```python
from build123d import *

# Parameters (mm, degrees)
SKICA1_W                                  = 49.2698
SKICA1_H                                  = 40
P_IDAT_VYSUNUT_M1_DEPTH                   = 2
ZKOSEN_1_SIZE                             = 0.5
SKICA4_W                                  = 63.2698
SKICA4_H                                  = 46
P_IDAT_VYSUNUT_M2_DEPTH                   = 2
KU_ELOV_ZAHLOUBEN_PRO_M3_ROUBU_SE_2_COUNT = 2
KU_ELOV_ZAHLOUBEN_PRO_M3_ROUBU_SE_2_PITCH = 66.661315559
F_3_4_3_4_PR_M_R_D_RY1_D                  = 3.4
F_3_4_3_4_PR_M_R_D_RY1_DEPTH              = 2
ODEBRAT_VYSUNUT_M1_DEPTH                  = 2
F_3_5_3_5_PR_M_R_D_RY1_D                  = 3.5
F_3_5_3_5_PR_M_R_D_RY1_DEPTH              = 4
F_4_5_4_5_PR_M_R_D_RY1_D                  = 4.5
F_4_5_4_5_PR_M_R_D_RY1_DEPTH              = 4
ZKOSEN_2_SIZE                             = 0.5


with BuildPart() as part:
    # Skica1 → Přidat vysunutím1 (new body)
    with BuildSketch(Plane.XY):
        with Locations((-294.244757855, 0)):
            Rectangle(SKICA1_W, SKICA1_H)
    extrude(amount=-P_IDAT_VYSUNUT_M1_DEPTH)

    # Zkosení1
    zkosen_1_edges = [part.edges().sort_by_distance(p)[0] for p in [
        (-269.609857855, 0, -2),
        (-294.244757855, 20, -2),
        (-318.879657855, 0, -2),
        (-294.244757855, -20, -2),
    ]]
    chamfer(zkosen_1_edges, length=ZKOSEN_1_SIZE)

    # Skica3 → Odebrat rotací2 (revolve, cut)
    with BuildSketch(Plane(origin=(0, -13.1125, 0), x_dir=(-1, 0, 0), z_dir=(0, -1, 0))):
        Polygon((273.341908662, 2), (276.609857855, 0.113248654), (276.609857855, 2), align=None)
    revolve(axis=Axis((-276.609857855, -13.1125, -0.113248654), (0, 0, -1)), mode=Mode.SUBTRACT)

    # Skica4 → Přidat vysunutím2 (add)
    with BuildSketch(Plane.XY):
        with Locations((-295.244757855, 0)):
            Rectangle(SKICA4_W, SKICA4_H)
    extrude(amount=P_IDAT_VYSUNUT_M2_DEPTH)

    # Skica7 → Kuželové zahloubení pro M3 šroubu se zápustnou hlavou plochou1 (revolve, cut)
    with BuildSketch(Plane(origin=(-321.879657855, -19, 2), x_dir=(0, -1, 0), z_dir=(1, 0, 0))):
        Polygon((0, 0), (0, 2), (1.6, 2), (1.6, 1.5), (3.1, 0), align=None)
    ku_elov_zahlouben_pro_m3_roubu_se_z_p = revolve(axis=Axis((-321.879657855, -19, 8.35), (0, 0, -1)), mode=Mode.SUBTRACT)

    # Ku_elov_ zahlouben_ pro M3 _roubu se 2: Kuželové zahloubení pro M3 šroubu se zápustnou hlavou plochou1 ×2
    with Locations(*[Vector(0.821612948, 0.570045756, 0) * (i * KU_ELOV_ZAHLOUBEN_PRO_M3_ROUBU_SE_2_PITCH) for i in range(1, KU_ELOV_ZAHLOUBEN_PRO_M3_ROUBU_SE_2_COUNT)]):
        add(ku_elov_zahlouben_pro_m3_roubu_se_z_p, mode=Mode.SUBTRACT)

    # Ø3.4 (3.4) průměr díry1
    with Locations(Plane(origin=(-267.109857855, -19, 2), x_dir=(1, 0, 0), z_dir=(0, 0, 1))):
        with Locations((0, 0), (-54.7698, 38)):
            Hole(F_3_4_3_4_PR_M_R_D_RY1_D / 2, depth=F_3_4_3_4_PR_M_R_D_RY1_DEPTH)

    # Skica9 → Odebrat vysunutím1 (cut)
    with BuildSketch(Plane.XY.offset(2)):
        with BuildLine():
            Line((-290.109857855, -14.1125), (-285.109857855, -14.1125))
            ThreePointArc((-285.109857855, -14.1125), (-284.109857855, -13.1125), (-285.109857855, -12.1125))
            Line((-285.109857855, -12.1125), (-290.109857855, -12.1125))
            ThreePointArc((-290.109857855, -12.1125), (-291.109857855, -13.1125), (-290.109857855, -14.1125))
        make_face()
        with BuildLine():
            Line((-277.609857855, 0.3875), (-277.609857855, -4.6125))
            ThreePointArc((-277.609857855, -4.6125), (-276.609857855, -5.6125), (-275.609857855, -4.6125))
            Line((-275.609857855, -4.6125), (-275.609857855, 0.3875))
            ThreePointArc((-275.609857855, 0.3875), (-276.609857855, 1.3875), (-277.609857855, 0.3875))
        make_face()
    extrude(amount=-ODEBRAT_VYSUNUT_M1_DEPTH, mode=Mode.SUBTRACT)

    # Ø3.5 (3.5) průměr díry1
    with Locations(Plane(origin=(-287.609857855, -13.1125, 2), x_dir=(1, 0, 0), z_dir=(0, 0, 1))):
        with Locations((0, 0), (11, 11)):
            Hole(F_3_5_3_5_PR_M_R_D_RY1_D / 2, depth=F_3_5_3_5_PR_M_R_D_RY1_DEPTH)

    # Ø4.5 (4.5) průměr díry1
    with Locations(Plane(origin=(-276.609857855, 8.8875, 2), x_dir=(1, 0, 0), z_dir=(0, 0, 1))):
        with Locations((0, 0), (-22, -22)):
            Hole(F_4_5_4_5_PR_M_R_D_RY1_D / 2, depth=F_4_5_4_5_PR_M_R_D_RY1_DEPTH)

    # Zkosení2
    zkosen_2_edges = [part.edges().sort_by_distance(p)[0] for p in [
        (-263.609857855, -23, 1),
        (-263.609857855, 23, 1),
        (-326.879657855, 23, 1),
        (-326.879657855, -23, 1),
    ]]
    chamfer(zkosen_2_edges, length=ZKOSEN_2_SIZE)


solid = part.part
```
Geometry: final body of the model. Coordinates: model frame, mm. A direction names the side the tool comes from. Coordinates: 2 decimals unless noted, no trailing zeros. Order: outer loops, then holes, each group sorted by start corner. A loop starts at its lowest first (then second) coordinate and runs counter-clockwise, first axis right, second up. Notation, with made-up numbers: (0, 75) -> (56, 75) arc R5 cw to (56, 81) -> close; hole circle Ø10 at (-19.75, 70). An arc over 180 degrees is marked (long way). Answer in a Markdown table with one row per item.
Item 1: Access query for faces 1 (the flat face through (-295, -20, -1)), 2 (the flat face through (-285, -13, 0)), 3 (the flat face through (-269.61, 0, -1)). Directions: +Z, -Z, +X, -X, +Y, -Y. A direction counts if a zero-diameter tool reaches every point of the face in a straight line with its end or side. Return the directions, or none.
Return value:
| item | result |
|---|---|
| face 1 | -Z, +X, -X, -Y |
| face 2 | +Z |
| face 3 | -Z, +X, +Y, -Y |
Item 2: Draft query along X for faces 4 (the cylindrical face through (-285.86, -13.04, -0.47)), 5 (the flat face through (-326.88, 0, 1)), 6 (the flat face through (-295, 0, -2)). Return one class per face: released by +X, released by -X, zero draft, split by the parting line, or undercut.
Return value:
| item | result |
|---|---|
| face 4 | undercut |
| face 5 | released by -X |
| face 6 | zero draft |
Item 3: Section A-A on x = -295. Output: boundary loops of the cut face in (y, z).
Return value:
| item | result |
|---|---|
| outline | (-23, 0) -> (-20, 0) -> (-20, -1.5) -> (-19.5, -2) -> (19.5, -2) -> (20, -1.5) -> (20, 0) -> (23, 0) -> (23, 2) -> (-23, 2) -> close |
Item 4: Ray query, L1, parallel to X at y = -14, z = 0.65; L2, parallel to Y at x = -276.5, z = -1.05; L3, parallel to X at y = -9, z = -0.3. Return the intervals inside material, ascending.
Return value:
| item | result |
|---|---|
| L1 | x = -326.88 to -300.68, -296.54 to -290.57, -284.65 to -263.61 |
| L2 | y = -20 to -14.73, -11.49 to -3.86, -0.37 to 6.64, 11.13 to 20 |
| L3 | x = -318.88 to -269.61 |
Item 5: Section B-B on y = 7.5. Output: boundary loops of the cut face in (x, z).
Return value:
| item | result |
|---|---|
| outline | (-326.88, 0) -> (-318.88, 0) -> (-318.88, -1.5) -> (-318.38, -2) -> (-278.38, -2) -> (-278.38, 2) -> (-326.88, 2) -> close; (-274.84, -2) -> (-270.11, -2) -> (-269.61, -1.5) -> (-269.61, 0) -> (-263.61, 0) -> (-263.61, 2) -> (-274.84, 2) -> close |
Item 6: Contact query for flat-ended pins moving along their axis: P1, Ø1.2, axis at y = 4, z = -1, coming from the +X side; P2, Ø2, axis at x = -285.5, y = -13, coming from the +Z side; P3, Ø0.8, axis at x = -299, z = -1, coming from the +Y side; P4, Ø5.5, axis at x = -321.88, y = 19, coming from the -Z side. Output: stop coordinate, or through.
Return value:
| item | result |
|---|---|
| P1 | stops at x = -269.61 |
| P2 | stops at z = 2 |
| P3 | stops at y = 20 |
| P4 | stops at z = 0 |
